from build123d import *

# Parameters (mm, degrees)
CHAMFER1_SIZE = 0.15
CHAMFER2_SIZE = 0.2


with BuildPart() as part:
    # Sketch1 → Base-Revolve (revolve)
    with BuildSketch(Plane.XY, mode=Mode.PRIVATE) as base_revolve_sk:
        with BuildLine():
            Line((0, 10), (-0.5, 10))
            Line((-0.5, 10), (-0.5, 6.2))
            Line((-0.5, 6.2), (-1.275, 6.2))
            Line((-1.275, 6.2), (-1.275, 2.757531755))
            Line((-1.275, 2.757531755), (-0.65, 0.425))
            Line((-0.65, 0.425), (-0.425, 0.2))
            Line((-0.425, 0.2), (-0.346410162, 0.2))
            ThreePointArc((-0.346410162, 0.2), (-0.2, 0.053589838), (0, 0))
            Line((0, 0), (0, 10))
        make_face()
    revolve(base_revolve_sk.sketch.rotate(Axis((0, -4.076789028, 0), (0, 1, 0)), 180), axis=Axis((0, -4.076789028, 0), (0, 1, 0)))

    # Chamfer1
    chamfer1_edges = [part.edges().sort_by_distance(p)[0] for p in [
        (-0.5, 10, 0),
    ]]
    chamfer(chamfer1_edges, length=CHAMFER1_SIZE)

    # Chamfer2
    chamfer2_edges = [part.edges().sort_by_distance(p)[0] for p in [
        (-1.275, 6.2, 0),
    ]]
    chamfer(chamfer2_edges, length=CHAMFER2_SIZE)


solid = part.part
Design review of the part built by this model. Coordinates are the model's own, in mm. A direction names the side the tool comes from. Coordinates: 2 decimals unless noted, no trailing zeros. Write each loop counter-clockwise with the first axis right and the second up, starting at its lowest first coordinate (ties: lowest second). Pieces come first, ordered by that corner, then holes. Notation, with made-up numbers: (65.5, -7.5) - (78.5, -7.5) arc R22 cw to (78.5, 22.5) - close; hole circle Ø10 at (17, 24). An arc over 180 degrees is marked (long way). One line per item, written item: value.
1) Add section A-A (x = 0). State the section outline as (y, z) points (3 decimals), plus the area to 3 significant figures.
Answer sheet:
outline: (0.2, -0.425) - (0.425, -0.65) - (2.758, -1.275) - (6, -1.275) - (6.2, -1.075) - (6.2, -0.5) - (9.85, -0.5) - (10, -0.35) - (10, 0.35) - (9.85, 0.5) - (6.2, 0.5) - (6.2, 1.075) - (6, 1.275) - (2.758, 1.275) - (0.425, 0.65) - (0.2, 0.425) - (0.2, 0.346) arc R0.4 ccw to (0.2, -0.346) - close
area: 17.3 mm2
2) To check wall thickness, follow probe 1 along X at (y, z) = (3.75, 0.15); probe 2 along Z at (x, y) = (-0.1, 7.5); probe 3 along X at (y, z) = (2.5, -0.4). State the ranges of each line that lie inside material, in increasing order.
Answer sheet:
probe 1: x = -1.27 to 1.27
probe 2: z = -0.49 to 0.49
probe 3: x = -1.14 to 1.14
3) Add section D-D (y = 5). State the section outline as (x, z) points (3 decimals).
Answer sheet:
outline: circle Ø2.55 at (0, 0)
4) Insertion check: pin 1 (1 mm diameter, centred on y = 5.5, z = 0.5, fed in from -X) (3 decimals); pin 2 (1 mm diameter, centred on x = 0, y = 9, fed in from +Z). Each pin has a flat end and moves straight along its axis. Give the tip position at first contact, or say it passes through.
Answer sheet:
pin 1: stops at x = -1.275
pin 2: stops at z = 0.5
5) For faces 1 (the face through (0.85, 1.32, -0.27)), 2 (the face through (-0.108, 7.999, 0.488)), list the 3-axis set-ups (+Z, -Z, +X, -X, +Y, -Y) from which the entire face can be reached by the end or side of a thin tool; tool diameter is ignored.
Answer sheet:
face 1: -Y
face 2: +Y
6) Add section B-B (z = 0). State the section outline as (x, y) points (3 decimals), plus the area to 3 significant figures.
Answer sheet:
outline: (-1.275, 2.758) - (-0.65, 0.425) - (-0.425, 0.2) - (-0.346, 0.2) arc R0.4 ccw to (0.346, 0.2) - (0.425, 0.2) - (0.65, 0.425) - (1.275, 2.758) - (1.275, 6) - (1.075, 6.2) - (0.5, 6.2) - (0.5, 9.85) - (0.35, 10) - (-0.35, 10) - (-0.5, 9.85) - (-0.5, 6.2) - (-1.075, 6.2) - (-1.275, 6) - close
area: 17.3 mm2
7) Add section C-C (y = 7.75). State the section outline as (x, z) points, plus the area to 3 significant figures.
Answer sheet:
outline: circle Ø1 at (0, 0)
area: 0.785 mm2
